Can you work these out from the model? Positions are in its coordinate system, mm. Round coordinates to 2 decimals unless told otherwise and drop trailing zeros. Loops run counter-clockwise (first coordinate to the right, second up) from the corner with the lowest first, then second, coordinate; pieces in that order, holes last.
(1) I want a section at D-D on x = -4. Write out the boundary of the cut face in (y, z).
(2) If I drill on line 1 along Z through (x, y) = (-9.25, 0.2); line 2 along X through (y, z) = (1.45, 4.25); line 3 along X through (y, z) = (0.4, -2), over which ranges is the centre line in solid material (lowest first)?
(3) I want a section at A-A on y = 1.5. Give the number of separate pieces and of enclosed holes in the cut face, plus the area to 3 significant figures.
(4) Will this pin go through, and if not, where does the flat tip stop? pin 1 Ø1.1 at (x, z) = (9.05, -4.81) entering from -Y.
(5) I want a section at B-B on x = 9. Write out the boundary of the cut face in (y, z).
(6) I want a section at C-C on z = -5.25. Write out the boundary of the cut face in (x, y), plus the area to 3 significant figures.
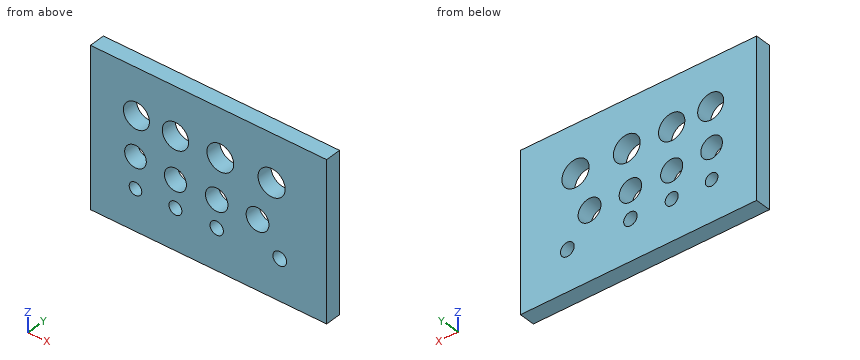
from build123d import *

# Parameters (mm, degrees)
SKETCH_1_W      = 30
SKETCH_1_H      = 20
SKETCH_1_R      = 0.8
SKETCH_1_R_2    = 0.825
SKETCH_1_R_3    = 0.85
SKETCH_1_R_4    = 0.875
SKETCH_1_R_5    = 1.375
SKETCH_1_R_6    = 1.4
SKETCH_1_R_7    = 1.425
SKETCH_1_R_8    = 1.45
SKETCH_1_R_9    = 1.65
SKETCH_1_R_10   = 1.675
SKETCH_1_R_11   = 1.7
SKETCH_1_R_12   = 1.725
EXTRUDE_1_DEPTH = 2


with BuildPart() as part:
    # 草图1 → 凸台-拉伸1 (new body)
    with BuildSketch(Plane(origin=(0, 0, 0), x_dir=(1, 0, 0), z_dir=(0, 1, 0))):
        Rectangle(SKETCH_1_W, SKETCH_1_H)
        with Locations((-9.279538905, 4.812680115)):
            Circle(SKETCH_1_R, mode=Mode.SUBTRACT)
        with Locations((-4.207492795, 4.812680115)):
            Circle(SKETCH_1_R_2, mode=Mode.SUBTRACT)
        with Locations((1.037463977, 4.812680115)):
            Circle(SKETCH_1_R_3, mode=Mode.SUBTRACT)
        with Locations((9.048991354, 4.812680115)):
            Circle(SKETCH_1_R_4, mode=Mode.SUBTRACT)
        with Locations((-9.279538905, 0.893371758)):
            Circle(SKETCH_1_R_5, mode=Mode.SUBTRACT)
        with Locations((-4.207492795, 1.354466859)):
            Circle(SKETCH_1_R_6, mode=Mode.SUBTRACT)
        with Locations((1.037463977, 1.354466859)):
            Circle(SKETCH_1_R_7, mode=Mode.SUBTRACT)
        with Locations((6.224783862, 1.354466859)):
            Circle(SKETCH_1_R_8, mode=Mode.SUBTRACT)
        with Locations((-9.161763858, -4.124789371)):
            Circle(SKETCH_1_R_9, mode=Mode.SUBTRACT)
        with Locations((-4.207492795, -3.948126801)):
            Circle(SKETCH_1_R_10, mode=Mode.SUBTRACT)
        with Locations((1.498559078, -3.948126801)):
            Circle(SKETCH_1_R_11, mode=Mode.SUBTRACT)
        with Locations((8.011527378, -3.948126801)):
            Circle(SKETCH_1_R_12, mode=Mode.SUBTRACT)
    extrude(amount=EXTRUDE_1_DEPTH)


solid = part.part
Filled sheet:
1. outline: (0, -10) - (2, -10) - (2, -5.61) - (0, -5.61) - close; (0, -4.01) - (2, -4.01) - (2, -2.74) - (0, -2.74) - close; (0, 0.03) - (2, 0.03) - (2, 2.29) - (0, 2.29) - close; (0, 5.61) - (2, 5.61) - (2, 10) - (0, 10) - close
2. line 1: z = -10 to -5.61, -4.01 to -2.27, 0.48 to 2.48, 5.77 to 10
2. line 2: x = -15 to -10.81, -7.52 to -5.86, -2.56 to -0.17, 3.17 to 6.31, 9.71 to 15
2. line 3: x = -15 to -10.1, -8.46 to -5.45, -2.97 to -0.23, 2.31 to 4.93, 7.52 to 15
3. separate pieces: 1
3. enclosed holes: 12
3. area: 530 mm2
4. pin 1: passes through
5. outline: (0, -10) - (2, -10) - (2, -5.69) - (0, -5.69) - close; (0, -3.94) - (2, -3.94) - (2, 2.53) - (0, 2.53) - close; (0, 5.36) - (2, 5.36) - (2, 10) - (0, 10) - close
6. outline: (-15, 0) - (-9.95, 0) - (-9.95, 2) - (-15, 2) - close; (-8.61, 0) - (-4.91, 0) - (-4.91, 2) - (-8.61, 2) - close; (-3.51, 0) - (0.31, 0) - (0.31, 2) - (-3.51, 2) - close; (1.77, 0) - (8.29, 0) - (8.29, 2) - (1.77, 2) - close; (9.81, 0) - (15, 0) - (15, 2) - (9.81, 2) - close
6. area: 48.6 mm2
